from build123d import *

# Parameters (mm, degrees)
SKETCH1_W                           = 10
SKETCH1_H                           = 13
EXTRUDE1_DEPTH                      = 3.175
SKETCH2_W                           = 8
SKETCH2_H                           = 8
EXTRUDE2_DEPTH                      = 3.5
F_0_80_TAPPED_HOLE1_D               = 1.19126
F_0_80_TAPPED_HOLE1_DEPTH           = 4
F_0_80_TAPPED_HOLE1_TIP             = 0.357890611
F_3_32_0_09375_DIAMETER_HOLE1_D     = 2.38125
F_3_32_0_09375_DIAMETER_HOLE1_DEPTH = 10
F_3_32_0_09375_DIAMETER_HOLE1_TIP   = 0.715399675
FILLET7_R                           = 1


with BuildPart() as part:
    # Sketch1 → Extrude1 (new body)
    with BuildSketch(Plane(origin=(0, 0, 0), x_dir=(1, 0, 0), z_dir=(0, 1, 0))):
        Rectangle(SKETCH1_W, SKETCH1_H)
    extrude(amount=EXTRUDE1_DEPTH)

    # Sketch2 → Extrude2 (cut)
    with BuildSketch(Plane(origin=(0, 3.175, 0), x_dir=(1, 0, 0), z_dir=(0, 1, 0))):
        with Locations((0, -1.5)):
            Rectangle(SKETCH2_W, SKETCH2_H)
    extrude(amount=-EXTRUDE2_DEPTH, mode=Mode.SUBTRACT)

    # #0-80 Tapped Hole1
    with Locations(Plane(origin=(0, 3.175, -4.5), x_dir=(0, 0, 1), z_dir=(0, 1, 0))):
        with Locations((0, 0)):
            Hole(F_0_80_TAPPED_HOLE1_D / 2, depth=F_0_80_TAPPED_HOLE1_DEPTH)
            with Locations((0, 0, -(F_0_80_TAPPED_HOLE1_DEPTH + F_0_80_TAPPED_HOLE1_TIP / 2))):  # 118° drill point
                Cone(0, F_0_80_TAPPED_HOLE1_D / 2, F_0_80_TAPPED_HOLE1_TIP, mode=Mode.SUBTRACT)

    # 3/32 (0.09375) Diameter Hole1
    with Locations(Plane(origin=(-3, 3.175, -4.5), x_dir=(0, 0, 1), z_dir=(0, 1, 0))):
        with Locations((0, 0), (0, 6)):
            Hole(F_3_32_0_09375_DIAMETER_HOLE1_D / 2, depth=F_3_32_0_09375_DIAMETER_HOLE1_DEPTH)
            with Locations((0, 0, -(F_3_32_0_09375_DIAMETER_HOLE1_DEPTH + F_3_32_0_09375_DIAMETER_HOLE1_TIP / 2))):  # 118° drill point
                Cone(0, F_3_32_0_09375_DIAMETER_HOLE1_D / 2, F_3_32_0_09375_DIAMETER_HOLE1_TIP, mode=Mode.SUBTRACT)

    # Fillet7
    fillet7_edges = [part.edges().sort_by_distance(p)[0] for p in [
        (-4, 1.5875, 5.5),
        (-4, 1.5875, -2.5),
        (4, 1.5875, -2.5),
        (4, 1.5875, 5.5),
        (-5, 1.5875, -6.5),
        (5, 1.5875, -6.5),
        (5, 1.5875, 6.5),
        (-5, 1.5875, 6.5),
    ]]
    fillet(fillet7_edges, radius=FILLET7_R)


solid = part.part
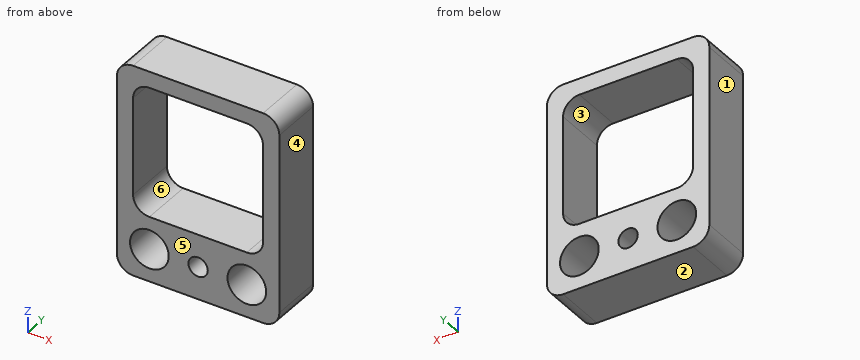
Source: CAD feature listing. Evaluate the final solid. Frame: model axes, mm. Face numbers are marked on the shaded views. A direction names the side the tool comes from. Round coordinates to 2 decimals unless told otherwise and drop trailing zeros. Write each loop counter-clockwise with the first axis right and the second up, starting at its lowest first coordinate (ties: lowest second). Pieces come first, ordered by that corner, then holes. Notation, with made-up numbers: M -1,61.25 L 51,61.25 A26 ccw 51,86.25 Z; hole C 36.25,-1.75 d4. An arc over 180 degrees is marked long. One line per item, written item: value. Start each with the question number.
Item 1: Mould query, pull axis X, two halves, no side actions, for the marked faces 1, 2, 3 and 4. Classes: pulls with the +X half, pulls with the -X half, needs draft (parallel to the pull), parting line crosses it, or undercut.
Item 2: Set-up query: the marked faces 5 and 6. Return all of +Z, -Z, +X, -X, +Y, -Y with unobstructed straight access to the full face (end or side cutting, diameter ignored); none if empty.
Item 3: Ray query, L1, parallel to X at y = 2.05, z = -4.5; L2, parallel to Z at x = -1.75, y = 2.2; L3, parallel to X at y = 1.4, z = 1. Return the intervals inside material, ascending. Write a range as from..to.
Item 4: Section query A-A (z = -1). Return the cut outline in (x, y) (3 decimals), plus the area to 3 significant figures.
Item 5: Section query D-D (y = 2.55). Return the cut outline in (x, z), plus the area to 3 significant figures.
Item 6: Section query B-B (x = 0). Return the cut outline in (y, z) (3 decimals).
Item 7: Section query C-C (z = -4.5). Return the cut outline in (x, y) (3 decimals), plus the area to 3 significant figures.
Result set:
1. face 1: pulls with the -X half
1. face 2: needs draft
1. face 3: undercut
1. face 4: pulls with the +X half
2. face 5: +Z, -Z, +X, -X, -Y
2. face 6: +Y, -Y
3. L1: x = -5..-4.19, -1.81..-0.6, 0.6..1.81, 4.19..5
3. L2: z = -6.5..-2.5, 5.5..6.5
3. L3: x = -5..-4, 4..5
4. outline: M -5,0 L -4,0 L -4,3.175 L -5,3.175 Z; M 4,0 L 5,0 L 5,3.175 L 4,3.175 Z
4. area: 6.35 mm²
5. outline: M -5,-5.5 A1 ccw -4,-6.5 L 4,-6.5 A1 ccw 5,-5.5 L 5,5.5 A1 ccw 4,6.5 L -4,6.5 A1 ccw -5,5.5 Z; hole C -3,-4.5 d2.38; hole M -4,-1.5 A1 ccw -3,-2.5 L 3,-2.5 A1 ccw 4,-1.5 L 4,4.5 A1 ccw 3,5.5 L -3,5.5 A1 ccw -4,4.5 Z; hole C 0,-4.5 d1.19; hole C 3,-4.5 d2.38
5. area: 56.0 mm²
6. outline: M 0,-6.5 L 3.175,-6.5 L 3.175,-5.096 L 0,-5.096 Z; M 0,-3.904 L 3.175,-3.904 L 3.175,-2.5 L 0,-2.5 Z; M 0,5.5 L 3.175,5.5 L 3.175,6.5 L 0,6.5 Z
7. outline: M -5,0 L -4.191,0 L -4.191,3.175 L -5,3.175 Z; M -1.809,0 L -0.596,0 L -0.596,3.175 L -1.809,3.175 Z; M 0.596,0 L 1.809,0 L 1.809,3.175 L 0.596,3.175 Z; M 4.191,0 L 5,0 L 5,3.175 L 4.191,3.175 Z
7. area: 12.8 mm²
